```python
from build123d import *

# Parameters (mm, degrees)
SKETCH2_W               = 256.44751275
SKETCH2_H               = 86.763856324
BOSS_EXTRUDE2_DEPTH     = 6
SKETCH5_W               = 8
SKETCH5_H               = 4.9
CUT_EXTRUDE7_DEPTH      = 1
CUT_EXTRUDE7_DEPTH_BACK = 7
FILLET1_R               = 10


with BuildPart() as part:
    # Sketch2 → Boss-Extrude2 (new body)
    with BuildSketch(Plane(origin=(0, 0, 0), x_dir=(1, 0, 0), z_dir=(0, 1, 0))):
        with Locations((-92.975357556, 78.4180884)):
            Rectangle(SKETCH2_W, SKETCH2_H)
    extrude(amount=BOSS_EXTRUDE2_DEPTH)

    # Sketch5 → Cut-Extrude7 (cut, two sides)
    with BuildSketch(Plane.XZ) as cut_extrude7_sk:
        with Locations((-203.05, -77.5)):
            Rectangle(SKETCH5_W, SKETCH5_H)
    extrude(amount=CUT_EXTRUDE7_DEPTH, mode=Mode.SUBTRACT)
    extrude(cut_extrude7_sk.sketch, amount=-CUT_EXTRUDE7_DEPTH_BACK, mode=Mode.SUBTRACT)

    # Fillet1
    fillet1_edges = [part.edges().sort_by_distance(p)[0] for p in [
        (35.248398819, 3, -35.036160238),
        (-221.199113931, 3, -35.036160238),
        (-221.199113931, 3, -121.800016562),
        (35.248398819, 3, -121.800016562),
    ]]
    fillet(fillet1_edges, radius=FILLET1_R)


solid = part.part
```
Part model, mm, in its own coordinate system. A direction names the side the tool comes from. Coordinates: 2 decimals unless noted, no trailing zeros. Write each loop counter-clockwise with the first axis right and the second up, starting at its lowest first coordinate (ties: lowest second). Pieces come first, ordered by that corner, then holes.
Item 1: Which spindle directions (+Z, -Z, +X, -X, +Y, -Y) get a long thin tool onto all of the face, cutting with end or side? Do faces 1 (the face through (-95, 0, -79)), 2 (the face through (-203, 3, -79.95)). Say none if no direction does.
Item 2: Probe line 1 (Z direction, x = -205, y = 5.1). List the from-to ranges inside material, lowest first.
Item 3: Mould opens along Z. For faces 3 (the face through (-221.199, 3, -78)), 4 (the face through (-207.05, 3, -78)), 5 (the face through (-95, 3, -121.8)) say: released by +Z, released by -Z, zero draft, split by the parting line, or undercut.
Item 4: Slice it at A-A (z = -77.5). Write the cut outline in (x, y), and give its area (3 significant figures).
Results found:
1. face 1: +Z, -Z, +X, -X, -Y
1. face 2: +Y, -Y
2. line 1: z = -121.8 to -79.95, -75.05 to -35.04
3. face 3: zero draft
3. face 4: undercut
3. face 5: released by -Z
4. outline: (-221.2, 0) - (-207.05, 0) - (-207.05, 6) - (-221.2, 6) - close; (-199.05, 0) - (35.25, 0) - (35.25, 6) - (-199.05, 6) - close
4. area: 1,490 mm2
